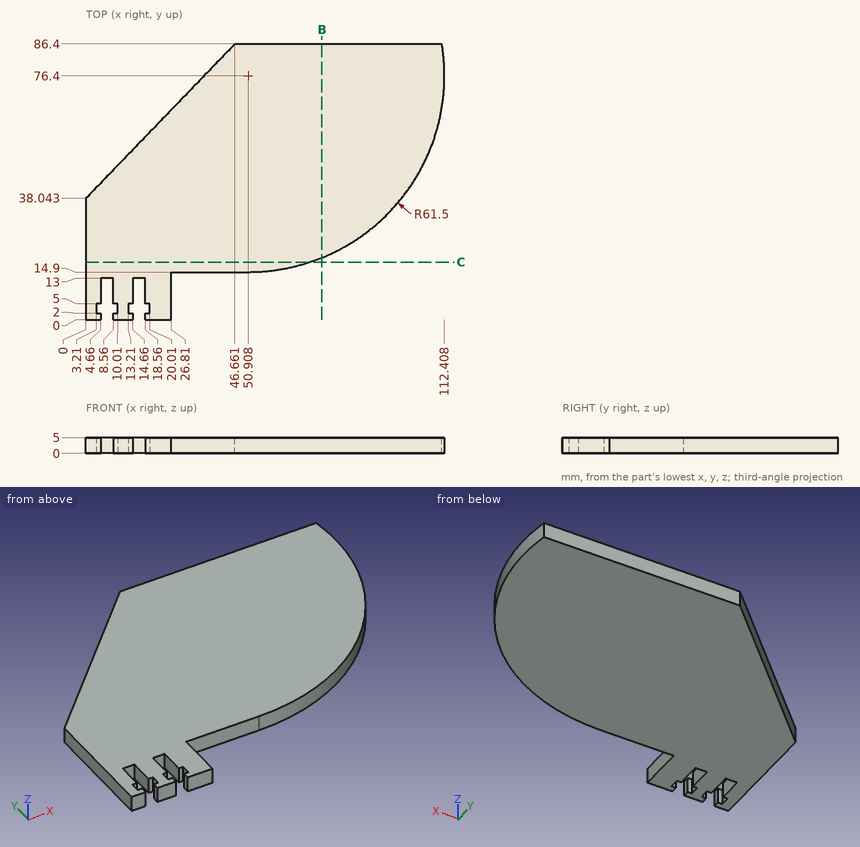
Print and shaded views of the part. All mm, measured from the part's lowest x, y and z. Round coordinates to 2 decimals unless told otherwise and drop trailing zeros. Write each loop counter-clockwise with the first axis right and the second up, starting at its lowest first coordinate (ties: lowest second). Pieces come first, ordered by that corner, then holes.
(1) Drop flat-ended pins along their axis: P1, Ø1.6, axis at x = 19, z = 2.5, coming from the +Y side; P2, Ø3, axis at x = 29, z = 4, coming from the -Y side; P3, Ø1.2, axis at x = 17, z = 2, coming from the -Y side. Give the stop position or say it passes through.
(2) Slice it at B-B, the plane x = 74. Write the cut outline in (y, z), and give its area (3 significant figures).
(3) Slice it at C-C, the plane y = 18. Write the cut outline in (x, z), and give its area (3 significant figures).
(4) Probe line 1 along X through (y, z) = (4, 4.45); line 2 along Y through (x, z) = (50, 2.4); line 3 along Y through (x, z) = (19.5, 1.05). List the from-to ranges inside material, lowest first.
From the geometry:
1. P1: stops at y = 58.56
1. P2: stops at y = 14.9
1. P3: stops at y = 13
2. outline: (19.4, 0) - (86.4, 0) - (86.4, 5) - (19.4, 5) - close
2. area: 335 mm2
3. outline: (0, 0) - (70.19, 0) - (70.19, 5) - (0, 5) - close
3. area: 351 mm2
4. line 1: x = 0 to 3.21, 10.01 to 13.21, 20.01 to 26.81
4. line 2: y = 14.9 to 86.4
4. line 3: y = 0 to 2, 5 to 58.25
